Geometry: final body of the model. Coordinates: model frame, mm. Coordinates: 2 decimals unless noted, no trailing zeros. Loops run counter-clockwise (first coordinate to the right, second up) from the corner with the lowest first, then second, coordinate; pieces in that order, holes last. Notation, with made-up numbers: (32, 37) -> (50, 37) arc R32 ccw to (50, 67) -> close; hole circle Ø2 at (66.25, 6.5). An arc over 180 degrees is marked (long way). One line per item, written item: value. Start each with the question number.
Item 1: Ray query, probe 1 along X at (y, z) = (3.25, 7); probe 2 along Y at (x, z) = (14, 1); probe 3 along Z at (x, y) = (22.5, 2.5). Return the intervals inside material, ascending. Write a range as from..to.
Item 2: Section query C-C on z = 18.5. Return loops of the section in (x, y).
Item 3: Contact query for flat-ended pins moving along their axis: pin 1 Ø1.8 at (x, y) = (-14, 0) entering from -Z; pin 2 Ø5 at (y, z) = (-1.5, 22) entering from +X; pin 3 Ø3 at (y, z) = (-2, 7.5) entering from -X. Output: stop coordinate, or through.
Item 4: Section query A-A on y = 3.25. Return loops of the section in (x, z).
Item 5: Section query B-B on x = -35. Return loops of the section in (y, z).
from build123d import *

# Parameters (mm, degrees)
SKETCH_1_W      = 210
SKETCH_1_H      = 10
SKETCH_1_R      = 1.5
EXTRUDE_1_DEPTH = 5
EXTRUDE_START   = 29
SKETCH_1_3_W    = 210
SKETCH_1_3_H    = 10
SKETCH_1_3_R    = 1.5
EXTRUDE_2_DEPTH = 5
SKETCH_1_4_W    = 3
SKETCH_1_4_H    = 10
EXTRUDE_3_DEPTH = 29


with BuildPart() as part:
    # Sketch 1 → Extrude 1 (new body)
    with BuildSketch(Plane.XY):
        Rectangle(SKETCH_1_W, SKETCH_1_H)
        with Locations((-70, 0)):
            Circle(SKETCH_1_R, mode=Mode.SUBTRACT)
        with Locations((-42, 0)):
            Circle(SKETCH_1_R, mode=Mode.SUBTRACT)
        with Locations((-14, 0)):
            Circle(SKETCH_1_R, mode=Mode.SUBTRACT)
        with Locations((14, 0)):
            Circle(SKETCH_1_R, mode=Mode.SUBTRACT)
        with Locations((42, 0)):
            Circle(SKETCH_1_R, mode=Mode.SUBTRACT)
        with Locations((70, 0)):
            Circle(SKETCH_1_R, mode=Mode.SUBTRACT)
    extrude(amount=EXTRUDE_1_DEPTH)



with BuildPart() as body_2:
    # Sketch 1_3 → Extrude 2 (new body)
    with BuildSketch(Plane.XY.offset(EXTRUDE_START)):
        Rectangle(SKETCH_1_3_W, SKETCH_1_3_H)
        with Locations((-70, 0)):
            Circle(SKETCH_1_3_R, mode=Mode.SUBTRACT)
        with Locations((-42, 0)):
            Circle(SKETCH_1_3_R, mode=Mode.SUBTRACT)
        with Locations((-14, 0)):
            Circle(SKETCH_1_3_R, mode=Mode.SUBTRACT)
        with Locations((14, 0)):
            Circle(SKETCH_1_3_R, mode=Mode.SUBTRACT)
        with Locations((42, 0)):
            Circle(SKETCH_1_3_R, mode=Mode.SUBTRACT)
        with Locations((70, 0)):
            Circle(SKETCH_1_3_R, mode=Mode.SUBTRACT)
    extrude(amount=EXTRUDE_2_DEPTH)


with BuildPart() as part_1:
    add(part.part)

    add(body_2.part)  # Extrude 3 merges body 2
    # Sketch 1_4 → Extrude 3 (add)
    with BuildSketch(Plane.XY):
        with Locations((-56, 0)):
            Rectangle(SKETCH_1_4_W, SKETCH_1_4_H)
        with Locations((-28, 0)):
            Rectangle(SKETCH_1_4_W, SKETCH_1_4_H)
        Rectangle(SKETCH_1_4_W, SKETCH_1_4_H)
        with Locations((28, 0)):
            Rectangle(SKETCH_1_4_W, SKETCH_1_4_H)
        with Locations((56, 0)):
            Rectangle(SKETCH_1_4_W, SKETCH_1_4_H)
    extrude(amount=EXTRUDE_3_DEPTH)


solid = part_1.part
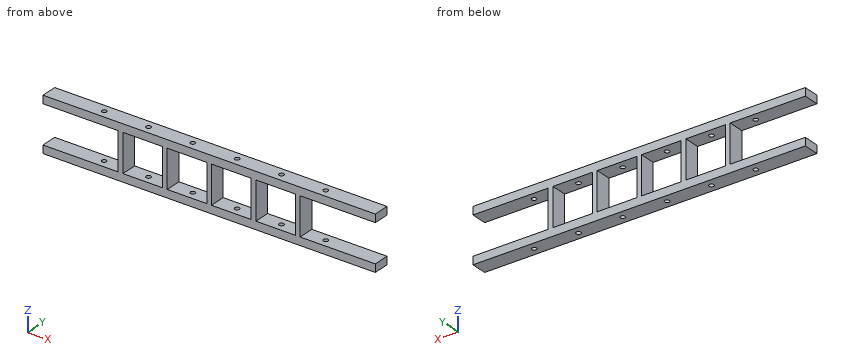
Reply:
1. probe 1: x = -57.5..-54.5, -29.5..-26.5, -1.5..1.5, 26.5..29.5, 54.5..57.5
1. probe 2: y = -5..-1.5, 1.5..5
1. probe 3: z = 0..5, 29..34
2. outline: (-57.5, -5) -> (-54.5, -5) -> (-54.5, 5) -> (-57.5, 5) -> close; (-29.5, -5) -> (-26.5, -5) -> (-26.5, 5) -> (-29.5, 5) -> close; (-1.5, -5) -> (1.5, -5) -> (1.5, 5) -> (-1.5, 5) -> close; (26.5, -5) -> (29.5, -5) -> (29.5, 5) -> (26.5, 5) -> close; (54.5, -5) -> (57.5, -5) -> (57.5, 5) -> (54.5, 5) -> close
3. pin 1: passes through
3. pin 2: stops at x = 57.5
3. pin 3: stops at x = -57.5
4. outline: (-105, 0) -> (105, 0) -> (105, 5) -> (57.5, 5) -> (57.5, 29) -> (105, 29) -> (105, 34) -> (-105, 34) -> (-105, 29) -> (-57.5, 29) -> (-57.5, 5) -> (-105, 5) -> close; hole (-54.5, 5) -> (-29.5, 5) -> (-29.5, 29) -> (-54.5, 29) -> close; hole (-26.5, 5) -> (-1.5, 5) -> (-1.5, 29) -> (-26.5, 29) -> close; hole (1.5, 5) -> (26.5, 5) -> (26.5, 29) -> (1.5, 29) -> close; hole (29.5, 5) -> (54.5, 5) -> (54.5, 29) -> (29.5, 29) -> close
5. outline: (-5, 0) -> (5, 0) -> (5, 5) -> (-5, 5) -> close; (-5, 29) -> (5, 29) -> (5, 34) -> (-5, 34) -> close
